Work out the finished part from the listing and answer in its coordinate system (mm). Face numbers are marked on the shaded views. A direction names the side the tool comes from. Round coordinates to 2 decimals unless told otherwise and drop trailing zeros. Order: outer loops, then holes, each group sorted by start corner. A loop starts at its lowest first (then second) coordinate and runs counter-clockwise, first axis right, second up. Notation, with made-up numbers: (15.5, -23) -> (49.5, -23) arc R32 ccw to (49.5, 11) -> close; hole circle Ø9 at (-0.75, 19). An arc over 180 degrees is marked (long way). Use a Markdown table: item, result. Add a question column.
Item 1: A cutting plane is placed at D-D, the plane y = -109. Determine the outline of the cut face in (x, z), plus the area to 3 significant figures.
Item 2: A tool of negligible diameter and unlimited length cuts with its end or side. For the marked faces 1, 2 and 3, from which of +Z, -Z, +X, -X, +Y, -Y can it reach the whole face along a straight path? Write none if from no direction.
Item 3: A cutting plane is placed at C-C, the plane z = 38. Determine the outline of the cut face in (x, y).
Item 4: Flat-ended cylindrical pins translate along their axes: P1, Ø4, axis at x = 119, z = -83.5, coming from the +Y side; P2, Ø12, axis at x = 80, z = -268, coming from the -Y side; P3, Ø18, axis at x = 33.5, y = -73, coming from the -Z side; P4, Ø17.5, axis at x = 0, z = -46.98, coming from the +Y side. Find the tip coordinate at first contact, or state that the pin passes through.
Item 5: A cutting plane is placed at A-A, the plane x = 0. Determine the outline of the cut face in (y, z), plus the area to 3 significant figures.
Item 6: A cutting plane is placed at B-B, the plane y = -74. Determine the outline of the cut face in (x, z), plus the area to 3 significant figures.
Item 7: Find the intervals of material crossed by L1, parallel to Z at x = 0, y = -35; L2, parallel to Y at x = 41, z = -124; L3, parallel to Y at x = 20, z = -205.5, in increasing order. Write a range as [from, to].
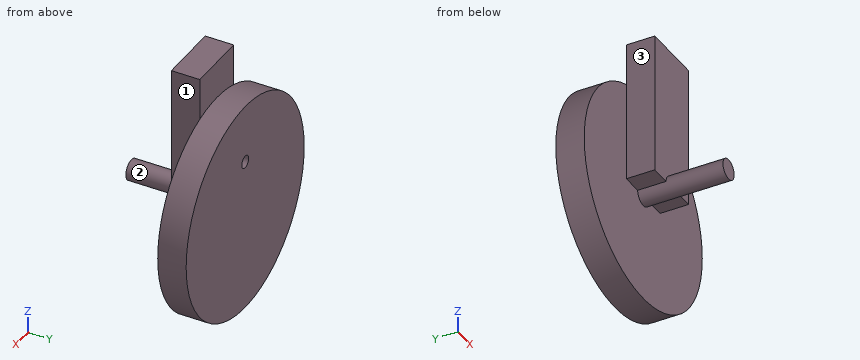
from build123d import *

# Parameters (mm, degrees)
F0_R     = 190.5
F1_DEPTH = 50.8
F2_R     = 11.061729
F3_DEPTH = 50.8
F4_W     = 109.096915
F4_H     = 254
F5_DEPTH = 50.8
F6_R     = 18.115742
F7_DEPTH = 152.4


with BuildPart() as f1:
    # F0 (on Front) → F1 (new body)
    with BuildSketch(Plane.XZ):
        with Locations((0, -132.514146)):
            Circle(F0_R)
    extrude(amount=F1_DEPTH)

    # F2 (on face) → F3 (cut)
    with BuildSketch(Plane.XZ.offset(50.8)):
        with Locations((0, -46.975374)):
            Circle(F2_R)
    extrude(amount=-F3_DEPTH, mode=Mode.SUBTRACT)

    # F4 (on face) → F5 (join)
    with BuildSketch(Plane.XZ.offset(50.8)):
        with Locations((-1e-06, -1.762878)):
            Rectangle(F4_W, F4_H)
    extrude(amount=F5_DEPTH)

    # F6 (on face) → F7 (join)
    with BuildSketch(Plane.XZ.offset(50.8)):
        with Locations((-2e-06, -128.762878)):
            Circle(F6_R)
    extrude(amount=F7_DEPTH)


solid = f1.part
Reported:
| question | item | result |
|---|---|---|
| 1 | outline | circle Ø36.23 at (0, -128.76) |
| 1 | area | 1,030 mm² |
| 2 | face 1 | +Z, -Z, +X, -Y |
| 2 | face 2 | -Y |
| 2 | face 3 | +Z, -Z, -X, -Y |
| 3 | outline | (-84.94, -50.8) -> (-54.55, -50.8) -> (-54.55, -101.6) -> (54.55, -101.6) -> (54.55, -50.8) -> (84.94, -50.8) -> (84.94, 0) -> (-84.94, 0) -> close |
| 4 | P1 | y = 0 |
| 4 | P2 | y = -50.8 |
| 4 | P3 | z = -128.76 |
| 4 | P4 | y = -50.8 |
| 5 | outline | (-203.2, -146.88) -> (-50.8, -146.88) -> (-50.8, -323.01) -> (0, -323.01) -> (0, -58.04) -> (-50.8, -58.04) -> (-50.8, -35.91) -> (0, -35.91) -> (0, 57.99) -> (-50.8, 57.99) -> (-50.8, 125.24) -> (-101.6, 125.24) -> (-101.6, -110.65) -> (-203.2, -110.65) -> close |
| 5 | area | 35,700 mm² |
| 6 | outline | (-54.55, -128.76) -> (-18.12, -128.76) arc R18.12 ccw to (18.12, -128.76) -> (54.55, -128.76) -> (54.55, 125.24) -> (-54.55, 125.24) -> close |
| 6 | area | 28,200 mm² |
| 7 | L1 | [-323.01, -58.04], [-35.91, 57.99] |
| 7 | L2 | [-101.6, 0] |
| 7 | L3 | [-50.8, 0] |
